Geometry check sheet. Reference: the model listing, model coordinates, mm. A direction names the side the tool comes from. Give positions to 0.01 mm unless a question says otherwise; leave off trailing zeros. Loops run counter-clockwise (first coordinate to the right, second up) from the corner with the lowest first, then second, coordinate; pieces in that order, holes last. Notation, with made-up numbers: (62.5, 15.25) -> (71.5, 15.25) arc R21 cw to (71.5, 23.25) -> close; hole circle Ø7 at (80, 9). An arc over 180 degrees is marked (long way). One line per question, with ' | ' between items.
from build123d import *

# Parameters (mm, degrees)
F0_R     = 26
F0_R_2   = 24
F1_DEPTH = 3.5
F0_R_3   = 22
F0_R_4   = 20
F2_DEPTH = 3.25
F3_SIZE  = 0.3


with BuildPart() as f1:
    # F0 (on Front) → F1 (new body, symmetric)
    with BuildSketch(Plane.XZ):
        Circle(F0_R)
        Circle(F0_R_2, mode=Mode.SUBTRACT)
    extrude(amount=F1_DEPTH, both=True)



with BuildPart() as f1b:
    # F0 (on Front) → F1, piece 2 (new body, symmetric)
    with BuildSketch(Plane.XZ):
        Circle(F0_R_3)
        Circle(F0_R_4, mode=Mode.SUBTRACT)
    extrude(amount=F1_DEPTH, both=True)


with BuildPart() as f1_1:
    add(f1.part)

    add(f1b.part)  # F2 merges F1b
    # F0 (on Front) → F2 (join, symmetric)
    with BuildSketch(Plane.XZ):
        Circle(F0_R_2)
        Circle(F0_R_3, mode=Mode.SUBTRACT)
    extrude(amount=F2_DEPTH, both=True)

    # F3
    f3_edges = [f1_1.edges().sort_by_distance(p)[0] for p in [
        (-26, -3.5, 0),
        (-26, 3.5, 0),
        (-20, -3.5, 0),
        (-20, 3.5, 0),
    ]]
    chamfer(f3_edges, length=F3_SIZE)


solid = f1_1.part
Item 1: Scan lines: probe 1 along Z at (x, y) = (0, -1); probe 2 along Z at (x, y) = (0, -3.4); probe 3 along X at (y, z) = (-1.25, -10.5). Record each from-to range of solid material in increasing order.
Result:
probe 1: -26 to -20, 20 to 26 | probe 2: -25.8 to -24, -22 to -20.2, 20.2 to 22, 24 to 25.8 | probe 3: -23.79 to -17.02, 17.02 to 23.79
Item 2: Release check for a two-part mould opening along X. For faces 1 (the face through (6.4, -3.5, -19.5)), 2 (the face through (-20.633, -0.045, -15.821)), 3 (the face through (-4.336, 0.045, -19.524)) record: pulls with the +X half, pulls with the -X half, needs draft (parallel to the pull), parting line crosses it, or undercut.
Result:
face 1: needs draft | face 2: parting line crosses it | face 3: undercut
Item 3: Sectioned sample at C-C (y = 1.5). Record the cut outline in (x, z), plus the area to 3 significant figures.
Result:
outline: circle Ø52 at (0, 0); hole circle Ø40 at (0, 0) | area: 867 mm2
Item 4: Set-up check for faces 4 (the face through (7, 3.25, -21.2)), 5 (the face through (7, -3.25, -21.2)), 6 (the face through (6.4, 3.5, -19.5)): record each of +Z, -Z, +X, -X, +Y, -Y from which the full face is reachable in a straight line by a thin tool's end or side.
Result:
face 4: +Y | face 5: -Y | face 6: +Z, -Z, +X, -X, +Y
